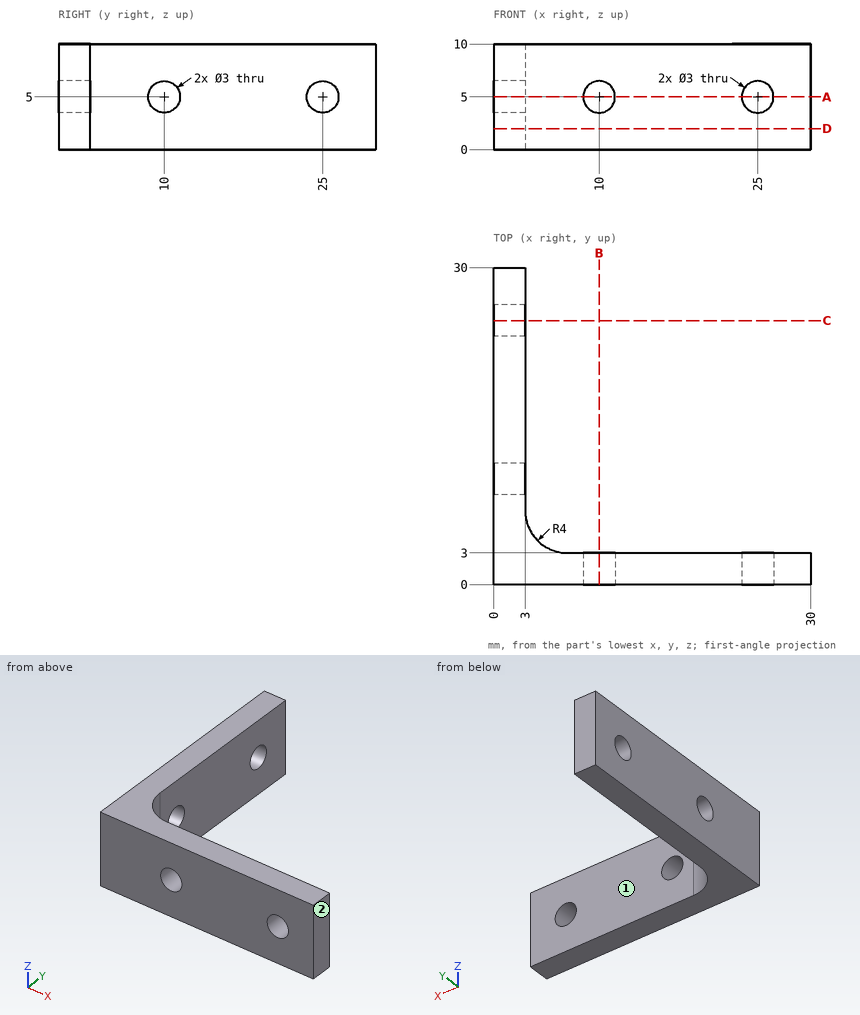
Design review of the part shown in the three views and the two pictorial views. Dimensions are in mm from the part's minimum x, y and z. A direction names the side the tool comes from. Coordinates: 2 decimals unless noted, no trailing zeros. Order: outer loops, then holes, each group sorted by start corner. A loop starts at its lowest first (then second) coordinate and runs counter-clockwise, first axis right, second up. Notation, with made-up numbers: (4.25, 7.25) - (33.25, 7.25) arc R19 cw to (33.25, 23.25) - close; hole circle Ø1 at (-3, 86.5). An arc over 180 degrees is marked (long way). Answer as CSV lines item,"result". Start each with the question number.
1) Add section D-D (z = 2). State the section outline as (x, y) points, then the cut area to 3 significant figures.
2) To check wall thickness, follow line 1 along Y through (x, z) = (1.4, 5); line 2 along Y through (x, z) = (16, 2.5). State the ranges of each line that lie inside material, in increasing order. Write a range as [from, to].
3) Machinability: for the marked faces 1 and 2, which of the approach directions +Z, -Z, +X, -X, +Y, -Y give a long, thin tool a straight path to every point of the face, cutting with its end or side? Answer none if there is none.
4) Add section A-A (z = 5). State the section outline as (x, y) points, then the cut area to 3 significant figures.
5) Insertion check: P1, Ø5, axis at y = 16.5, z = 4, coming from the -X side; P2, Ø2.5, axis at y = 10, z = 5, coming from the +X side; P3, Ø3.5, axis at x = 25, z = 5, coming from the +Y side; P4, Ø1.5, axis at y = 13, z = 3.5, coming from the +X side. Each pin has a flat end and moves straight along its axis. Give the tip position at first contact, or say it passes through.
6) Add section B-B (x = 10). State the section outline as (y, z) points.
Result:
1,outline,"(0, 0) - (30, 0) - (30, 3) - (7, 3) arc R4 cw to (3, 7) - (3, 30) - (0, 30) - close"
1,area,"174 mm^2"
2,line 1,"[0, 8.5], [11.5, 23.5], [26.5, 30]"
2,line 2,"[0, 3]"
3,face 1,"+Z, -Z, +X, +Y"
3,face 2,"+Z, -Z, +X, +Y, -Y"
4,outline,"(0, 0) - (8.5, 0) - (8.5, 3) - (7, 3) arc R4 cw to (3, 7) - (3, 8.5) - (0, 8.5) - close; (0, 11.5) - (3, 11.5) - (3, 23.5) - (0, 23.5) - close; (0, 26.5) - (3, 26.5) - (3, 30) - (0, 30) - close; (11.5, 0) - (23.5, 0) - (23.5, 3) - (11.5, 3) - close; (26.5, 0) - (30, 0) - (30, 3) - (26.5, 3) - close"
4,area,"138 mm^2"
5,P1,"x = 0"
5,P2,"through"
5,P3,"y = 3"
5,P4,"x = 3"
6,outline,"(0, 0) - (3, 0) - (3, 3.5) - (0, 3.5) - close; (0, 6.5) - (3, 6.5) - (3, 10) - (0, 10) - close"
